from build123d import *

# Parameters (mm, degrees)
SKETCH2_R                = 6.5
SIX_DRAINAGE_HOLES_DEPTH = 373.86056375


with BuildPart() as part:
    # Sketch1 → Planter Body + Central Socket (revolve)
    with BuildSketch(Plane.XY, mode=Mode.PRIVATE) as planter_body_central_socket_sk:
        Polygon((0, 0), (130, 0), (130, 10), (162, 10), (162, 0), (170, 0), (170, 12), (148, 30), (160, 280), (156, 285), (152, 280), (143, 18), (100, 18), (30, 80), (30, 100), (13.5, 100), (13.5, 8), (0, 8), align=None)
    revolve(planter_body_central_socket_sk.sketch.rotate(Axis((0, -10, 0), (0, 1, 0)), 90), axis=Axis((0, -10, 0), (0, 1, 0)))

    # Sketch2 → Six Drainage Holes (cut, through all)
    with BuildSketch(Plane(origin=(0, 0, 0), x_dir=(1, 0, 0), z_dir=(0, 1, 0))):
        with Locations(Location((118, 0, 0), (0, 0, 270))):
            Circle(SKETCH2_R)
        with Locations(Location((59, 102.190997647, 0), (0, 0, 270))):
            Circle(SKETCH2_R)
        with Locations(Location((-59, 102.190997647, 0), (0, 0, 270))):
            Circle(SKETCH2_R)
        with Locations(Location((-118, 0, 0), (0, 0, 270))):
            Circle(SKETCH2_R)
        with Locations(Location((-59, -102.190997647, 0), (0, 0, 270))):
            Circle(SKETCH2_R)
        with Locations(Location((59, -102.190997647, 0), (0, 0, 270))):
            Circle(SKETCH2_R)
    extrude(amount=SIX_DRAINAGE_HOLES_DEPTH, mode=Mode.SUBTRACT)


solid = part.part
Geometry: final body of the model. Coordinates: model frame, mm. A direction names the side the tool comes from. Coordinates: 2 decimals unless noted, no trailing zeros. Order: outer loops, then holes, each group sorted by start corner. A loop starts at its lowest first (then second) coordinate and runs counter-clockwise, first axis right, second up.
1) Ray query, probe 1 along X at (y, z) = (4, 0); probe 2 along X at (y, z) = (30, 0); probe 3 along X at (y, z) = (13.5, 0). Return the intervals inside material, ascending.
Result sheet:
probe 1: x = -170 to -162, -130 to -124.5, -111.5 to 111.5, 124.5 to 130, 162 to 170
probe 2: x = -148 to -143.41, -86.45 to -13.5, 13.5 to 86.45, 143.41 to 148
probe 3: x = -168.17 to -124.5, -111.5 to -13.5, 13.5 to 111.5, 124.5 to 168.17
2) Set-up query: faces 1 (the cylindrical face through (-39.048, 5.07, -123.997)), 2 (the conical face through (-44.78, 29.13, -142.18)), 3 (the cylindrical face through (-51.06, 6.08, -162.15)), 4 (the cylindrical face through (-25.296, 90.14, -16.128)), 5 (the flat face through (62, 0, 150)). Return all of +Z, -Z, +X, -X, +Y, -Y with unobstructed straight access to the full face (end or side cutting, diameter ignored); none if empty.
Result sheet:
face 1: -Y
face 2: none
face 3: +Y, -Y
face 4: +Y
face 5: +Z, -Z, +X, -X, -Y
3) First-contact query: P1, Ø6, axis at x = 96, z = 92.5, coming from the -Y side; P2, Ø6, axis at x = 101.5, y = 33.5, coming from the -Z side; P3, Ø1.5, axis at y = 191.5, z = -105.5, coming from the +X side; P4, Ø10.5, axis at x = 118, z = 0, coming from the +Y side. Flat tips, straight axial feed; report the tip coordinate or a pass-through.
Result sheet:
P1: stops at y = 10
P2: stops at z = -110.69
P3: stops at x = 115.27
P4: passes through
4) Draft query along X for faces 6 (the conical face through (-152.773, 156.75, 20.059)), 7 (the flat face through (13, 100, -6)), 8 (the flat face through (-2, 0, -2)). Return one class per face: released by +X, released by -X, zero draft, split by the parting line, or undercut.
Result sheet:
face 6: split by the parting line
face 7: undercut
face 8: zero draft
5) Section C-C (y = 134). Return loops of the section in (x, z), then the cut area to 3 significant figures.
Result sheet:
outline: circle Ø305.98 at (0, 0); hole circle Ø293.97 at (0, 0)
area: 5,660 mm2
6) Section D-D (x = 59). Give the number of separate pieces and of enclosed holes in the cut face, then the cut area to 3 significant figures.
Result sheet:
separate pieces: 3
enclosed holes: 0
area: 12,000 mm2
7) Section B-B (y = 85). Return loops of the section in (x, z), then the cut area to 3 significant figures.
Result sheet:
outline: circle Ø301.28 at (0, 0); circle Ø60 at (0, 0); hole circle Ø290.6 at (0, 0); hole circle Ø27 at (0, 0)
area: 7,220 mm2
